```python
from build123d import *

# Parameters (mm, degrees)
SKETCH_1_W         = 10
SKETCH_1_H         = 10
EXTRUDE_1_DEPTH    = 3
HOLE_WIZARD_M3_1_D = 2.5
HOLE_WIZARD_M3_2_D = 2.5
HOLE_WIZARD_M3_3_D = 2.5
FILLET_1_R         = 1
CHAMFER_1_SIZE     = 0.2


with BuildPart() as part:
    # 草图1 → 凸台-拉伸1 (new, symmetric)
    with BuildSketch(Plane(origin=(0, 0, 0), x_dir=(1, 0, 0), z_dir=(0, 1, 0))):
        Rectangle(SKETCH_1_W, SKETCH_1_H)
    extrude(amount=EXTRUDE_1_DEPTH, both=True)

    # M3 螺纹孔1 (through all)
    with Locations(Plane(origin=(0, 3, 0), x_dir=(1, 0, 0), z_dir=(0, 1, 0))):
        with Locations((0, 0)):
            Hole(HOLE_WIZARD_M3_1_D / 2)

    # M3 螺纹孔2 (through all)
    with Locations(Plane.XY.offset(5)):
        with Locations((0, 0)):
            Hole(HOLE_WIZARD_M3_2_D / 2)

    # M3 螺纹孔3 (through all)
    with Locations(Plane(origin=(5, 0, 0), x_dir=(0, 0, -1), z_dir=(1, 0, 0))):
        with Locations((0, 0)):
            Hole(HOLE_WIZARD_M3_3_D / 2)

    # 圆角1
    fillet_1_edges = [part.edges().sort_by_distance(p)[0] for p in [
        (5, 0, 5),
        (-5, 0, 5),
        (-5, 0, -5),
        (5, 0, -5),
    ]]
    fillet(fillet_1_edges, radius=FILLET_1_R)

    # 倒角1
    chamfer_1_edges = [part.edges().sort_by_distance(p)[0] for p in [
        (0, -3, -5),
        (0, 3, -5),
        (5, -3, 0),
        (0, -3, 5),
        (-5, -3, 0),
        (-4.707106781, -3, -4.707106781),
        (-4.707106781, -3, 4.707106781),
        (4.707106781, -3, 4.707106781),
        (4.707106781, -3, -4.707106781),
        (5, 3, 0),
        (-5, 3, 0),
        (0, 3, 5),
        (-4.707106781, 3, -4.707106781),
        (-4.707106781, 3, 4.707106781),
        (4.707106781, 3, 4.707106781),
        (4.707106781, 3, -4.707106781),
    ]]
    chamfer(chamfer_1_edges, length=CHAMFER_1_SIZE)


solid = part.part
```
CAD build for the part. Positions are in the model's coordinates, mm. Round coordinates to 2 decimals unless told otherwise and drop trailing zeros. Write each loop counter-clockwise with the first axis right and the second up, starting at its lowest first coordinate (ties: lowest second). Pieces come first, ordered by that corner, then holes. Notation, with made-up numbers: (63.5, 2) - (92.5, 2) arc R16 ccw to (92.5, 7) - close; hole circle Ø3 at (1.5, 22). An arc over 180 degrees is marked (long way). Write item = value, one per line. Start each with the question number.
Q1. Mould opens along Z. For faces 1 (the flat face through (1, 3, -1)), 2 (the cylindrical face through (-0.577, 2.162, 1.109)), 3 (the flat face through (-1, 1, 5)) say: pulls with the +Z half, pulls with the -Z half, needs draft (parallel to the pull), parting line crosses it, or undercut.
Q2. Band-saw the part on B-B (z = 0). Give the cut face in (x, y), then the cut area to 3 significant figures.
Q3. Band-saw the part on C-C (x = 2). Give the cut face in (y, z).
Q4. Drop a flat-ended pin along its axis: pin 1 (2 mm diameter, centred on x = 0, z = 0, fed in from +Y). Give the stop position or say it passes through.
Q5. Probe L1, parallel to Z at x = 0, y = -2.5; L2, parallel to Y at x = 1.9, z = 0; L3, parallel to Z at x = 0.5, y = 2. List the from-to ranges inside material, lowest first. Write a range as from..to.
Q6. Band-saw the part on A-A (x = 0). Give the cut face in (y, z), then the cut area to 3 significant figures.
Q7. Band-saw the part on D-D (z = 1.5). Give the cut face in (x, y), then the cut area to 3 significant figures.
Answers below:
q1.face_1 = needs draft
q1.face_2 = undercut
q1.face_3 = pulls with the +Z half
q2.outline = (-5, -2.8) - (-4.8, -3) - (-1.25, -3) - (-1.25, -1.25) - (-5, -1.25) - close; (-5, 1.25) - (-1.25, 1.25) - (-1.25, 3) - (-4.8, 3) - (-5, 2.8) - close; (1.25, -3) - (4.8, -3) - (5, -2.8) - (5, -1.25) - (1.25, -1.25) - close; (1.25, 1.25) - (5, 1.25) - (5, 2.8) - (4.8, 3) - (1.25, 3) - close
q2.area = 26.2 mm2
q3.outline = (-3, -4.8) - (-2.8, -5) - (2.8, -5) - (3, -4.8) - (3, 4.8) - (2.8, 5) - (-2.8, 5) - (-3, 4.8) - close; hole circle Ø2.5 at (0, 0)
q4.pin_1 = through
q5.L1 = -5..-1.25, 1.25..5
q5.L2 = -3..-1.25, 1.25..3
q5.L3 = -5..-1.15, 1.15..5
q6.outline = (-3, -4.8) - (-2.8, -5) - (-1.25, -5) - (-1.25, -1.25) - (-3, -1.25) - close; (-3, 1.25) - (-1.25, 1.25) - (-1.25, 5) - (-2.8, 5) - (-3, 4.8) - close; (1.25, -5) - (2.8, -5) - (3, -4.8) - (3, -1.25) - (1.25, -1.25) - close; (1.25, 1.25) - (3, 1.25) - (3, 4.8) - (2.8, 5) - (1.25, 5) - close
q6.area = 26.2 mm2
q7.outline = (-5, -2.8) - (-4.8, -3) - (4.8, -3) - (5, -2.8) - (5, 2.8) - (4.8, 3) - (-4.8, 3) - (-5, 2.8) - close; hole circle Ø2.5 at (0, 0)
q7.area = 55.0 mm2
